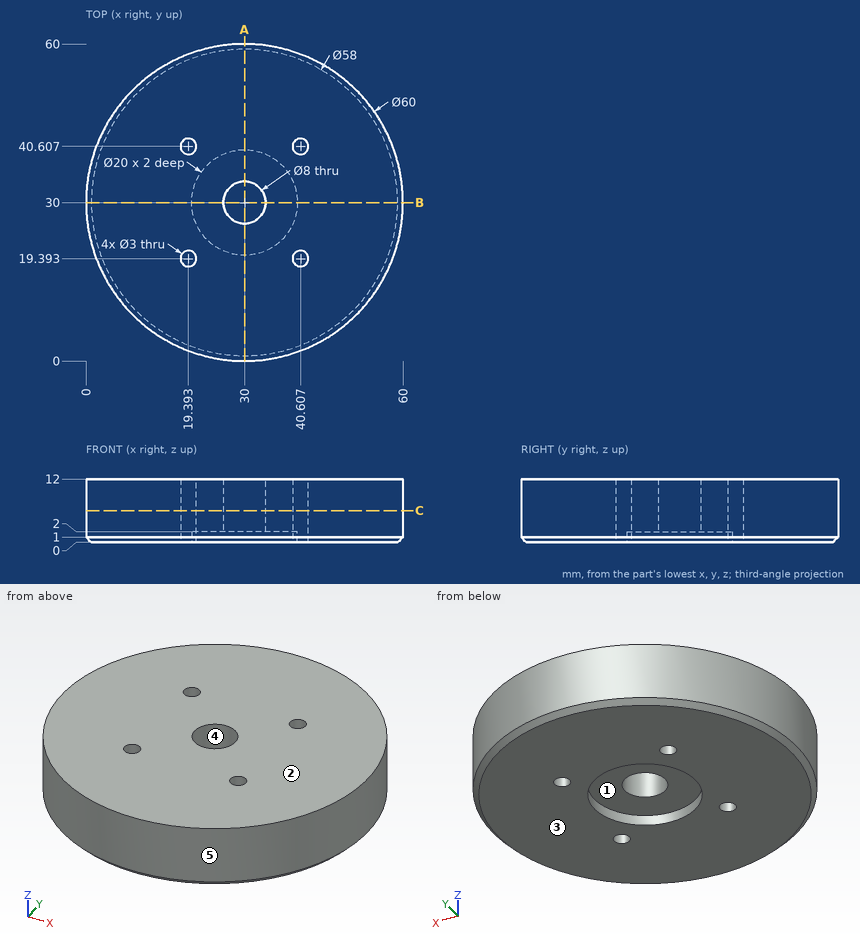
Geometry check sheet. Reference: drawing and pictorial views, mm from the part's lowest x, y, z. A direction names the side the tool comes from. Give positions to 0.01 mm unless a question says otherwise; leave off trailing zeros. Order: outer loops, then holes, each group sorted by start corner. A loop starts at its lowest first (then second) coordinate and runs counter-clockwise, first axis right, second up. Notation, with made-up numbers: M 0,33.5 L 6,33.5 A10 cw 6,45.5 Z; hole C -5,62.25 d2. An arc over 180 degrees is marked long. Answer as CSV lines item,"result". Start each with the question number.
Item 1: Gauge pin test, flat ends, axial feed: P1, Ø2.5, axis at x = 40.61, y = 40.61, coming from the +Z side; P2, Ø4, axis at y = 8, z = 2, coming from the -X side; P3, Ø5, axis at x = 13.5, z = 5, coming from the +Y side; P4, Ø3, axis at x = 42, z = 5.5, coming from the +Y side. Record the tip position at first contact, or that the pin passes through.
Item 2: Cross-section at A-A on x = 30. Enter the section's corners in (y, z), plus the area to 3 significant figures.
Item 3: Tool access check on the marked faces 1 and 2. Record the directions out of +Z, -Z, +X, -X, +Y, -Y that give a thin tool (end or side, any length) a straight path to the whole face; none if there is none.
Item 4: Cross-section at C-C on z = 6. Enter the section's corners in (x, y), plus the area to 3 significant figures.
Item 5: Mould release check, pull along X, two halves, no side actions. Record for the marked faces 3, 4 and 5: +X half, -X half, draft (parallel to the pull), parting line (faces both ways), or undercut.
Item 6: Thickness scan on line 1 (Y direction, x = 30, z = 1.55); line 2 (Y direction, x = 30, z = 8.5); line 3 (X direction, y = 41.5, z = 10). Record the ranges inside material, lowest first. Write a range as [from, to].
Established:
1,P1,"passes through"
1,P2,"stops at x = 7.64"
1,P3,"stops at y = 56.53"
1,P4,"stops at y = 58.1"
2,outline,"M 0,1 L 1,0 L 20,0 L 20,2 L 26,2 L 26,12 L 0,12 Z; M 34,2 L 40,2 L 40,0 L 59,0 L 60,1 L 60,12 L 34,12 Z"
2,area,"599 mm^2"
3,face 1,"-Z"
3,face 2,"+Z, +X, -X, +Y, -Y"
4,outline,"C 30,30 d60; hole C 19.39,19.39 d3; hole C 19.39,40.61 d3; hole C 30,30 d8; hole C 40.61,19.39 d3; hole C 40.61,40.61 d3"
4,area,"2,750 mm^2"
5,face 3,"draft"
5,face 4,"undercut"
5,face 5,"parting line"
6,line 1,"y = [0, 20], [40, 60]"
6,line 2,"y = [0, 26], [34, 60]"
6,line 3,"x = [2.29, 18.19], [20.6, 39.4], [41.81, 57.71]"
